```python
from build123d import *

# Parameters (mm, degrees)
SKETCH1_R           = 66.3575
BOSS_EXTRUDE1_DEPTH = 5.08
CUT_EXTRUDE1_REACH  = 95.981
SKETCH3_R           = 19.05
CUT_EXTRUDE2_REACH  = 95.981
SKETCH3_4_R         = 3.900616975
SKETCH3_4_W         = 5.08
SKETCH3_4_H         = 59.193573399


with BuildPart() as part:
    # Sketch1 → Boss-Extrude1 (new body)
    with BuildSketch(Plane.XY):
        Circle(SKETCH1_R)
    extrude(amount=BOSS_EXTRUDE1_DEPTH)

    # Sketch3 → Cut-Extrude1 (cut, up to next)
    with BuildSketch(Plane.XY, mode=Mode.PRIVATE) as cut_extrude1_sk1:
        Circle(SKETCH3_R)
    cut_extrude1_tool1 = extrude(cut_extrude1_sk1.sketch, amount=CUT_EXTRUDE1_REACH, mode=Mode.PRIVATE) & part.part
    add(cut_extrude1_tool1.solids().sort_by_distance((0, 0, 0))[0], mode=Mode.SUBTRACT)

    # Sketch3_4 → Cut-Extrude2 (cut, up to next)
    with BuildSketch(Plane.XY, mode=Mode.PRIVATE) as cut_extrude2_sk1:
        with BuildLine():
            Line((-50.832794134, -42.65377881), (-41.104029707, -34.490376167))
            ThreePointArc((-41.104029707, -34.490376167), (-50.4215568, -18.35194584), (-53.6575, 0))
            Line((-53.6575, 0), (-66.3575, 0))
            ThreePointArc((-66.3575, 0), (-62.355653084, -22.695601661), (-50.832794134, -42.65377881))
        make_face()
    cut_extrude2_tool1 = extrude(cut_extrude2_sk1.sketch, amount=CUT_EXTRUDE2_REACH, mode=Mode.PRIVATE) & part.part
    # Sketch3_4 → Cut-Extrude2 (cut, up to next)
    with BuildSketch(Plane.XY, mode=Mode.PRIVATE) as cut_extrude2_sk2:
        with BuildLine():
            ThreePointArc((50.832794134, 42.65377881), (62.355653084, 22.695601661), (66.3575, 0))
            Line((66.3575, 0), (53.6575, 0))
            ThreePointArc((53.6575, 0), (50.4215568, 18.35194584), (41.104029707, 34.490376167))
            Line((41.104029707, 34.490376167), (50.832794134, 42.65377881))
        make_face()
    cut_extrude2_tool2 = extrude(cut_extrude2_sk2.sketch, amount=CUT_EXTRUDE2_REACH, mode=Mode.PRIVATE) & part.part
    # Sketch3_4 → Cut-Extrude2 (cut, up to next)
    with BuildSketch(Plane.XY, mode=Mode.PRIVATE) as cut_extrude2_sk3:
        with Locations((10.33807752, -50.8)):
            Circle(SKETCH3_4_R)
    cut_extrude2_tool3 = extrude(cut_extrude2_sk3.sketch, amount=CUT_EXTRUDE2_REACH, mode=Mode.PRIVATE) & part.part
    # Sketch3_4 → Cut-Extrude2 (cut, up to next)
    with BuildSketch(Plane.XY, mode=Mode.PRIVATE) as cut_extrude2_sk4:
        with Locations((-9.98192248, -50.8)):
            Circle(SKETCH3_4_R)
    cut_extrude2_tool4 = extrude(cut_extrude2_sk4.sketch, amount=CUT_EXTRUDE2_REACH, mode=Mode.PRIVATE) & part.part
    # Sketch3_4 → Cut-Extrude2 (cut, up to next)
    with BuildSketch(Plane.XY, mode=Mode.PRIVATE) as cut_extrude2_sk5:
        with Locations(Location((10.33807752, 50.8, 0), (0, 0, 180))):
            Circle(SKETCH3_4_R)
    cut_extrude2_tool5 = extrude(cut_extrude2_sk5.sketch, amount=CUT_EXTRUDE2_REACH, mode=Mode.PRIVATE) & part.part
    # Sketch3_4 → Cut-Extrude2 (cut, up to next)
    with BuildSketch(Plane.XY, mode=Mode.PRIVATE) as cut_extrude2_sk6:
        with Locations(Location((-9.98192248, 50.8, 0), (0, 0, 180))):
            Circle(SKETCH3_4_R)
    cut_extrude2_tool6 = extrude(cut_extrude2_sk6.sketch, amount=CUT_EXTRUDE2_REACH, mode=Mode.PRIVATE) & part.part
    # Sketch3_4 → Cut-Extrude2 (cut, up to next)
    with BuildSketch(Plane.XY, mode=Mode.PRIVATE) as cut_extrude2_sk7:
        with Locations((0.17807752, -38.26186151)):
            Rectangle(SKETCH3_4_W, SKETCH3_4_H)
    cut_extrude2_tool7 = extrude(cut_extrude2_sk7.sketch, amount=CUT_EXTRUDE2_REACH, mode=Mode.PRIVATE) & part.part
    add(cut_extrude2_tool1.solids().sort_by_distance((-55.456661, -20.184574, 0))[0], mode=Mode.SUBTRACT)
    add(cut_extrude2_tool2.solids().sort_by_distance((55.456661, 20.184574, 0))[0], mode=Mode.SUBTRACT)
    add(cut_extrude2_tool3.solids().sort_by_distance((10.338078, -50.8, 0))[0], mode=Mode.SUBTRACT)
    add(cut_extrude2_tool4.solids().sort_by_distance((-9.981922, -50.8, 0))[0], mode=Mode.SUBTRACT)
    add(cut_extrude2_tool5.solids().sort_by_distance((10.338078, 50.8, 0))[0], mode=Mode.SUBTRACT)
    add(cut_extrude2_tool6.solids().sort_by_distance((-9.981922, 50.8, 0))[0], mode=Mode.SUBTRACT)
    add(cut_extrude2_tool7.solids().sort_by_distance((0.178078, -38.261862, 0))[0], mode=Mode.SUBTRACT)


solid = part.part
```
CAD build for the part. Positions are in the model's coordinates, mm. A direction names the side the tool comes from. Coordinates: 2 decimals unless noted, no trailing zeros. Write each loop counter-clockwise with the first axis right and the second up, starting at its lowest first coordinate (ties: lowest second). Pieces come first, ordered by that corner, then holes. Notation, with made-up numbers: (39.25, 15) -> (73.25, 15) arc R17 ccw to (73.25, 39) -> close; hole circle Ø5 at (-33, 54). An arc over 180 degrees is marked (long way). Return JSON: item names as keys, results as strings. Group by question number.
Q1. Cut at D-D, the plane y = -27.5. Give the cut face in (x, z).
Q2. Cut at A-A, the plane z = 0.9. State how many separate pieces and enclosed holes the cut face has, then the cut area to 3 significant figures.
Q3. Drill centre lines: line 1 (X direction, y = -50.8, z = 3.75); line 2 (Y direction, x = -12, z = 2.55); line 3 (X direction, y = -50.5, z = 2.55). Where is each one in solid material? Low to high.
Q4. Cut at B-B, the plane x = -9. Give the cut face in (y, z) (3 decimals), then the cut area to 3 significant figures.
Q5. Which spindle directions (+Z, -Z, +X, -X, +Y, -Y) get a long thin tool onto all of the face, cutting with end or side? Do faces 4 (the face through (-60, 0, 3)), 5 (the face through (2.718, -43, 3)), 6 (the face through (9.83, -46.933, 2.504)), 7 (the face through (45.9, 38.515, 2.504)), 8 (the face through (-46, -38.6, 2.5)). Say none if no direction does.
Q6. Pull direction X, two halves, no side cores. Call faces 1 (the face through (60, 0, 3)), 2 (the face through (0.62, 19.04, 2.5)), 3 (the face through (-50.33, -18.6, 2.5)): released by +X, released by -X, zero draft, split by the parting line, or undercut.
Q7. Cut at C-C, the plane y = 50.8. Give the cut face in (x, z).
Q8. Flat gauge pins, fed straight in: pin 1 (10 mm diameter, centred on x = -9.98, y = -50.8, fed in from -Z); pin 2 (2 mm diameter, centred on x = 13.5, z = 2.5, fed in from -Y); pin 3 (2.5 mm diameter, centred on x = 59, z = 3.5, fed in from +Y); pin 4 (1.5 mm diameter, centred on x = -59.5, z = 1.5, fed in from -Y). Where does each tip first touch, or does it go through?
Returned:
{
 "1": {"outline": "(-46.07, 0) -> (-2.36, 0) -> (-2.36, 5.08) -> (-46.07, 5.08) -> close; (2.72, 0) -> (60.39, 0) -> (60.39, 5.08) -> (2.72, 5.08) -> close"},
 "2": {"separate pieces": "1", "enclosed holes": "4", "area": "11,200 mm2"},
 "3": {"line 1": "x = -42.69 to -13.88, -6.08 to -2.36, 2.72 to 6.44, 14.24 to 42.69", "line 2": "y = -65.26 to -54.14, -47.46 to -14.8, 14.8 to 47.46, 54.14 to 65.26", "line 3": "x = -43.05 to -13.87, -6.09 to -2.36, 2.72 to 6.45, 14.23 to 43.05"},
 "4": {"outline": "(-65.744, 0) -> (-54.575, 0) -> (-54.575, 5.08) -> (-65.744, 5.08) -> close; (-47.025, 0) -> (-16.79, 0) -> (-16.79, 5.08) -> (-47.025, 5.08) -> close; (16.79, 0) -> (47.025, 0) -> (47.025, 5.08) -> (16.79, 5.08) -> close; (54.575, 0) -> (65.744, 0) -> (65.744, 5.08) -> (54.575, 5.08) -> close", "area": "421 mm2"},
 "5": {"face 4": "+Z, -Z, -X, -Y", "face 5": "+Z, -Z, -Y", "face 6": "+Z, -Z", "face 7": "+Z, -Z, +X", "face 8": "+Z, -Z, -X"},
 "6": {"face 1": "zero draft", "face 2": "undercut", "face 3": "released by -X"},
 "7": {"outline": "(-42.69, 0) -> (-13.88, 0) -> (-13.88, 5.08) -> (-42.69, 5.08) -> close; (-6.08, 0) -> (6.44, 0) -> (6.44, 5.08) -> (-6.08, 5.08) -> close; (14.24, 0) -> (42.69, 0) -> (42.69, 5.08) -> (14.24, 5.08) -> close"},
 "8": {"pin 1": "stops at z = 0", "pin 2": "stops at y = -65.17", "pin 3": "stops at y = 0", "pin 4": "stops at y = 0"}
}
